Check sheet for the modelled part. Datum: model origin and axes. Units: mm. Face numbers are marked on the shaded views. A direction names the side the tool comes from. Coordinates: 2 decimals unless noted, no trailing zeros. Loops run counter-clockwise (first coordinate to the right, second up) from the corner with the lowest first, then second, coordinate; pieces in that order, holes last. Notation, with made-up numbers: M 45,-14.75 L 60,-14.75 A35 ccw 60,22.25 Z; hole C -33.5,81 d10. An arc over 180 degrees is marked long. Write each question's results on one line, items separated by ' | '. Start each with the question number.
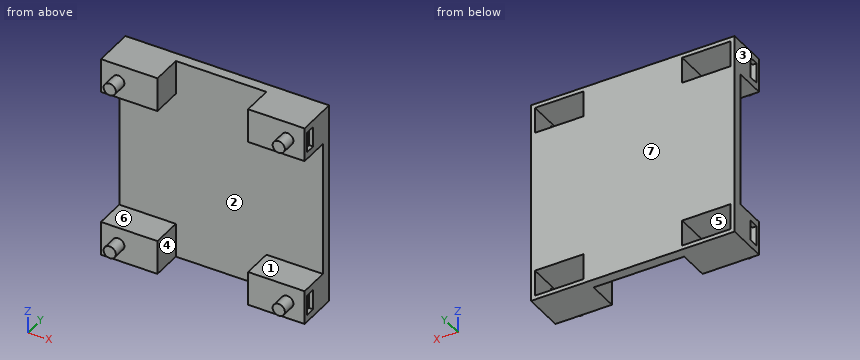
from build123d import *

# Parameters (mm, degrees)
BOSS_EXTRUDE1_DEPTH      = 2
BOSS_EXTRUDE1_DEPTH_BACK = 3
SKETCH1_W                = 100
SKETCH1_H                = 100
SKETCH3_W                = 27.75
SKETCH3_H                = 16.75
BOSS_EXTRUDE4_DEPTH      = 18
SKETCH4_W                = 23.75
SKETCH4_H                = 12.75
CUT_EXTRUDE1_DEPTH       = 18
SKETCH5_R                = 3
BOSS_EXTRUDE5_DEPTH      = 7
SKETCH6_W                = 10
SKETCH6_H                = 5
CUT_EXTRUDE2_DEPTH       = 2
SKETCH7_W                = 10
SKETCH7_H                = 5
CUT_EXTRUDE3_DEPTH       = 2


with BuildPart() as part:
    # Sketch1 → Boss-Extrude1 (new, two sides: drawn at the far end of the back side and taken through both)
    with BuildSketch(Plane(origin=(0, 0, 0), x_dir=(1, 0, 0), z_dir=(0, 1, 0)).offset(-BOSS_EXTRUDE1_DEPTH_BACK)):
        Rectangle(SKETCH1_W, SKETCH1_H)
    extrude(amount=BOSS_EXTRUDE1_DEPTH + BOSS_EXTRUDE1_DEPTH_BACK)

    # Sketch3 → Boss-Extrude4 (add)
    with BuildSketch(Plane(origin=(0, 0, 0), x_dir=(1, 0, 0), z_dir=(0, 1, 0))):
        with Locations((-36.125, -41.625)):
            Rectangle(SKETCH3_W, SKETCH3_H)
        with Locations((36.125, -41.625)):
            Rectangle(SKETCH3_W, SKETCH3_H)
        with Locations((36.125, 41.625)):
            Rectangle(SKETCH3_W, SKETCH3_H)
        with Locations((-36.125, 41.625)):
            Rectangle(SKETCH3_W, SKETCH3_H)
    extrude(amount=-BOSS_EXTRUDE4_DEPTH)

    # Sketch4 → Cut-Extrude1 (cut)
    with BuildSketch(Plane(origin=(0, 2, 0), x_dir=(1, 0, 0), z_dir=(0, 1, 0))):
        with Locations((-36.125, -41.625)):
            Rectangle(SKETCH4_W, SKETCH4_H)
        with Locations((36.125, -41.625)):
            Rectangle(SKETCH4_W, SKETCH4_H)
        with Locations((36.125, 41.625)):
            Rectangle(SKETCH4_W, SKETCH4_H)
        with Locations((-36.125, 41.625)):
            Rectangle(SKETCH4_W, SKETCH4_H)
    extrude(amount=-CUT_EXTRUDE1_DEPTH, mode=Mode.SUBTRACT)

    # Sketch5 → Boss-Extrude5 (add)
    with BuildSketch(Plane(origin=(0, -18, 0), x_dir=(-1, 0, 0), z_dir=(0, -1, 0))):
        with Locations(Location((41.5, -41.625, 0), (0, 0, 90))):
            Circle(SKETCH5_R)
        with Locations(Location((-41.5, -41.625, 0), (0, 0, 270))):
            Circle(SKETCH5_R)
        with Locations(Location((41.5, 41.625, 0), (0, 0, 270))):
            Circle(SKETCH5_R)
        with Locations(Location((-41.5, 41.625, 0), (0, 0, 270))):
            Circle(SKETCH5_R)
    extrude(amount=BOSS_EXTRUDE5_DEPTH)

    # Sketch6 → Cut-Extrude2 (cut)
    with BuildSketch(Plane(origin=(50, 0, 0), x_dir=(0, 0, -1), z_dir=(1, 0, 0))):
        with Locations((-41.625, -13.5)):
            Rectangle(SKETCH6_W, SKETCH6_H)
        with Locations((41.625, -13.5)):
            Rectangle(SKETCH6_W, SKETCH6_H)
    extrude(amount=-CUT_EXTRUDE2_DEPTH, mode=Mode.SUBTRACT)

    # Sketch7 → Cut-Extrude3 (cut)
    with BuildSketch(Plane.ZY.offset(50)):
        with Locations((41.625, -13.5)):
            Rectangle(SKETCH7_W, SKETCH7_H)
        with Locations((-41.625, -13.5)):
            Rectangle(SKETCH7_W, SKETCH7_H)
    extrude(amount=-CUT_EXTRUDE3_DEPTH, mode=Mode.SUBTRACT)


solid = part.part
1) Release check for a two-part mould opening along X. For the marked faces 1, 2 and 3 record: +X half, -X half, draft (parallel to the pull), parting line (faces both ways), or undercut.
2) Section check B-B (x = 41.5). Enter the section's corners in (y, z) (3 decimals).
3) Section check A-A (y = -4.5). Give the number of separate pieces and of enclosed holes in the cut face, then the cut area to 3 significant figures.
4) Thickness scan on probe 1 along X at (y, z) = (-6, 37.5); probe 2 along Z at (x, y) = (39.5, 0.75); probe 3 along Z at (x, y) = (35.5, -10). Record the ranges inside material, lowest first.
5) Set-up check for the marked faces 4, 5, 6 and 7: record each of +Z, -Z, +X, -X, +Y, -Y from which the full face is reachable in a straight line by a thin tool's end or side.
6) Section check C-C (x = 31). Enter the section's corners in (y, z), then the cut area to 4 significant figures.
7) Gauge pin test, flat ends, axial feed: P1, Ø0.6, axis at x = -49, z = -43.5, coming from the -Y side; P2, Ø1, axis at x = -1.5, z = -4, coming from the -Y side. Record the tip position at first contact, or that the pin passes through.
Return value:
1) face 1: draft | face 2: undercut | face 3: -X half
2) outline: M -25,-44.625 L -18,-44.625 L -18,-50 L 2,-50 L 2,-48 L -16,-48 L -16,-35.25 L 2,-35.25 L 2,35.25 L -16,35.25 L -16,48 L 2,48 L 2,50 L -18,50 L -18,44.625 L -25,44.625 L -25,38.625 L -18,38.625 L -18,33.25 L -3,33.25 L -3,-33.25 L -18,-33.25 L -18,-38.625 L -25,-38.625 Z
3) separate pieces: 4 | enclosed holes: 4 | area: 648 mm2
4) probe 1: x = -50 to -48, -24.25 to -22.25, 22.25 to 24.25, 48 to 50 | probe 2: z = -50 to -48, -35.25 to 35.25, 48 to 50 | probe 3: z = -50 to -48, -35.25 to -33.25, 33.25 to 35.25, 48 to 50
5) face 4: +Z, -Z, -Y | face 5: +Y | face 6: +X, -X, -Y | face 7: +Z, -Z, +X, -X, +Y
6) outline: M -18,-50 L 2,-50 L 2,-48 L -16,-48 L -16,-35.25 L 2,-35.25 L 2,35.25 L -16,35.25 L -16,48 L 2,48 L 2,50 L -18,50 L -18,33.25 L -3,33.25 L -3,-33.25 L -18,-33.25 Z | area: 543.5 mm2
7) P1: stops at y = -18 | P2: stops at y = -3
